Geometry check sheet. Reference: the model listing, model coordinates, mm. Face numbers are marked on the shaded views. Round coordinates to 2 decimals unless told otherwise and drop trailing zeros. Loops run counter-clockwise (first coordinate to the right, second up) from the corner with the lowest first, then second, coordinate; pieces in that order, holes last. Notation, with made-up numbers: (62, 48.5) -> (118, 48.5) arc R17 cw to (118, 70.5) -> close; hole circle Ø11 at (-35.5, 61). An arc over 180 degrees is marked (long way). Use a Markdown table: item, result. Add a question column.
Q1. Material ranges on L1, parallel to Y at x = 26, z = 5; L2, parallel to Y at x = 22, z = 6.25; L3, parallel to Y at x = 16, z = 0.75, recorded low to high.
Q2. Sectioned sample at D-D, the plane x = 11. Enter the section's corners in (y, z).
Q3. Sectioned sample at C-C, the plane y = -13. Enter the section's corners in (x, z).
Q4. Sectioned sample at A-A, the plane x = 0. Enter the section's corners in (y, z).
Q5. Gauge pin test, flat ends, axial feed: P1, Ø3.5, axis at x = 0, z = 4, coming from the +Y side; P2, Ø2.5, axis at x = -0.5, z = 3.5, coming from the -Y side; P3, Ø6, axis at x = -23.08, y = -23.08, coming from the +Z side. Record the tip position at first contact, or that the pin passes through.
Q6. Release check for a two-part mould opening along X. For the marked faces 1 and 2 record: released by +X, released by -X, zero draft, split by the parting line, or undercut.
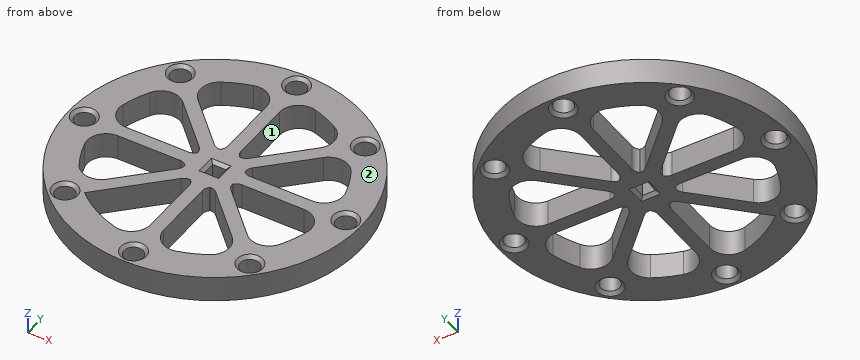
```python
from build123d import *

# Parameters (mm, degrees)
SKETCH1_R           = 36.449
SKETCH1_W           = 3.302
SKETCH1_H           = 3.302
SKETCH1_R_2         = 2.38125
BOSS_EXTRUDE1_DEPTH = 6.35
FILLET1_R           = 4.7625
FILLET2_R           = 2.38125
CHAMFER1_SIZE       = 0.79375


with BuildPart() as part:
    # Sketch1 → Boss-Extrude1 (new body)
    with BuildSketch(Plane.XY):
        Circle(SKETCH1_R)
        with BuildLine():
            Line((-1.651, 28.781685844), (-1.651, 6.131614714))
            ThreePointArc((-1.651, 6.131614714), (-2.430039796, 5.866635031), (-3.168273048, 5.50313964))
            Line((-3.168273048, 5.50313964), (-19.184291938, 21.51915853))
            ThreePointArc((-19.184291938, 21.51915853), (-11.032380672, 26.634523043), (-1.651, 28.781685844))
        make_face(mode=Mode.SUBTRACT)
        with BuildLine():
            Line((-21.51915853, 19.184291938), (-5.50313964, 3.168273048))
            ThreePointArc((-5.50313964, 3.168273048), (-5.866635031, 2.430039796), (-6.131614714, 1.651))
            Line((-6.131614714, 1.651), (-28.781685844, 1.651))
            ThreePointArc((-28.781685844, 1.651), (-26.634523043, 11.032380672), (-21.51915853, 19.184291938))
        make_face(mode=Mode.SUBTRACT)
        with BuildLine():
            Line((-28.781685844, -1.651), (-6.131614714, -1.651))
            ThreePointArc((-6.131614714, -1.651), (-5.866635031, -2.430039796), (-5.50313964, -3.168273048))
            Line((-5.50313964, -3.168273048), (-21.51915853, -19.184291938))
            ThreePointArc((-21.51915853, -19.184291938), (-26.634523043, -11.032380672), (-28.781685844, -1.651))
        make_face(mode=Mode.SUBTRACT)
        with BuildLine():
            Line((-19.184291938, -21.51915853), (-3.168273048, -5.50313964))
            ThreePointArc((-3.168273048, -5.50313964), (-2.430039796, -5.866635031), (-1.651, -6.131614714))
            Line((-1.651, -6.131614714), (-1.651, -28.781685844))
            ThreePointArc((-1.651, -28.781685844), (-11.032380672, -26.634523043), (-19.184291938, -21.51915853))
        make_face(mode=Mode.SUBTRACT)
        with BuildLine():
            Line((1.651, -28.781685844), (1.651, -6.131614714))
            ThreePointArc((1.651, -6.131614714), (2.430039796, -5.866635031), (3.168273048, -5.50313964))
            Line((3.168273048, -5.50313964), (19.184291938, -21.51915853))
            ThreePointArc((19.184291938, -21.51915853), (11.032380672, -26.634523043), (1.651, -28.781685844))
        make_face(mode=Mode.SUBTRACT)
        with BuildLine():
            Line((21.51915853, -19.184291938), (5.50313964, -3.168273048))
            ThreePointArc((5.50313964, -3.168273048), (5.866635031, -2.430039796), (6.131614714, -1.651))
            Line((6.131614714, -1.651), (28.781685844, -1.651))
            ThreePointArc((28.781685844, -1.651), (26.634523043, -11.032380672), (21.51915853, -19.184291938))
        make_face(mode=Mode.SUBTRACT)
        with BuildLine():
            Line((28.781685844, 1.651), (6.131614714, 1.651))
            ThreePointArc((6.131614714, 1.651), (5.866635031, 2.430039796), (5.50313964, 3.168273048))
            Line((5.50313964, 3.168273048), (21.51915853, 19.184291938))
            ThreePointArc((21.51915853, 19.184291938), (26.634523043, 11.032380672), (28.781685844, 1.651))
        make_face(mode=Mode.SUBTRACT)
        with BuildLine():
            Line((19.184291938, 21.51915853), (3.168273048, 5.50313964))
            ThreePointArc((3.168273048, 5.50313964), (2.430039796, 5.866635031), (1.651, 6.131614714))
            Line((1.651, 6.131614714), (1.651, 28.781685844))
            ThreePointArc((1.651, 28.781685844), (11.032380672, 26.634523043), (19.184291938, 21.51915853))
        make_face(mode=Mode.SUBTRACT)
        Rectangle(SKETCH1_W, SKETCH1_H, mode=Mode.SUBTRACT)
        with Locations((-23.079258231, -23.079258231)):
            Circle(SKETCH1_R_2, mode=Mode.SUBTRACT)
        with Locations((-32.639, 0)):
            Circle(SKETCH1_R_2, mode=Mode.SUBTRACT)
        with Locations((0, -32.639)):
            Circle(SKETCH1_R_2, mode=Mode.SUBTRACT)
        with Locations((23.079258231, -23.079258231)):
            Circle(SKETCH1_R_2, mode=Mode.SUBTRACT)
        with Locations((-23.079258231, 23.079258231)):
            Circle(SKETCH1_R_2, mode=Mode.SUBTRACT)
        with Locations((23.079258231, 23.079258231)):
            Circle(SKETCH1_R_2, mode=Mode.SUBTRACT)
        with Locations((0, 32.639)):
            Circle(SKETCH1_R_2, mode=Mode.SUBTRACT)
        with Locations((32.639, 0)):
            Circle(SKETCH1_R_2, mode=Mode.SUBTRACT)
    extrude(amount=BOSS_EXTRUDE1_DEPTH)

    # Fillet1
    fillet1_edges = [part.edges().sort_by_distance(p)[0] for p in [
        (21.51915853, 19.184291938, 3.175),
        (28.781685844, 1.651, 3.175),
        (19.184291938, 21.51915853, 3.175),
        (1.651, 28.781685844, 3.175),
        (-1.651, 28.781685844, 3.175),
        (-19.184291938, 21.51915853, 3.175),
        (-21.51915853, 19.184291938, 3.175),
        (-28.781685844, 1.651, 3.175),
        (-28.781685844, -1.651, 3.175),
        (-21.51915853, -19.184291938, 3.175),
        (-1.651, -28.781685844, 3.175),
        (1.651, -28.781685844, 3.175),
        (19.184291938, -21.51915853, 3.175),
        (21.51915853, -19.184291938, 3.175),
        (28.781685844, -1.651, 3.175),
    ]]
    fillet(fillet1_edges, radius=FILLET1_R)

    # Fillet2
    # the kernel refuses this fillet: 2.38125 mm, written as the material it adds along each edge
    with BuildSketch(Plane(origin=(6.131614714, -1.651, 0), x_dir=(-0.36304434778587014, -0.931771861316241, 0), z_dir=(0, 0, 1)), Plane(origin=(1.651, 6.131614714, 0), x_dir=(0.9317718613162208, -0.36304434778592154, 0), z_dir=(0, 0, 1)), Plane(origin=(5.50313964, 3.168273048, 0), x_dir=(0.40215108146465606, -0.9155733218463759, 0), z_dir=(0, 0, 1)), Plane(origin=(-6.131614714, 1.651, 0), x_dir=(0.3630443477859294, 0.9317718613162179, 0), z_dir=(0, 0, 1))) as fillet2_piece_1:
        with BuildLine():
            CenterArc((1.633270214, 2.367244602), FILLET2_R, 201.287277983, 62.495506179)
            Line((-0.585511531, 1.502745249), (0, 0))
            ThreePointArc((0, 0), (0.687692722, 0.037347727), (1.375385443, 0))
        make_face()
    extrude(amount=6.35)
    with BuildSketch(Plane(origin=(5.50313964, -3.168273048, 0), x_dir=(0.7071067811865454, -0.7071067811865497, 0), z_dir=(0, 0, 1)), Plane(origin=(3.168273048, 5.50313964, 0), x_dir=(0.7071067811865503, 0.7071067811865448, 0), z_dir=(0, 0, 1)), Plane(origin=(6.131614714, 1.651, 0), x_dir=(1, 0, 0), z_dir=(0, 0, 1)), Plane(origin=(-1.651, 6.131614714, 0), x_dir=(0, 1, 0), z_dir=(0, 0, 1)), Plane(origin=(-5.50313964, 3.168273048, 0), x_dir=(-0.7071067811865499, 0.7071067811865452, 0), z_dir=(0, 0, 1)), Plane(origin=(-6.131614714, -1.651, 0), x_dir=(-1, 0, 0), z_dir=(0, 0, 1)), Plane(origin=(1.651, -6.131614714, 0), x_dir=(0, -1, 0), z_dir=(0, 0, 1))) as fillet2_piece_2:
        with BuildLine():
            CenterArc((1.61278239, 2.38125), FILLET2_R, 207.504493821, 62.495506179)
            ThreePointArc((-0.499325911, 1.281545455), (-0.214863395, 0.654331608), (0, 0))
            Line((0, 0), (1.61278239, 0))
        make_face()
    extrude(amount=6.35)
    with BuildSketch(Plane(origin=(3.168273048, -5.50313964, 0), x_dir=(0.7071067811865439, -0.7071067811865511, 0), z_dir=(0, 0, 1)), Plane(origin=(-3.168273048, 5.50313964, 0), x_dir=(-0.7071067811865503, 0.7071067811865448, 0), z_dir=(0, 0, 1)), Plane(origin=(-5.50313964, -3.168273048, 0), x_dir=(-0.7071067811865455, -0.7071067811865496, 0), z_dir=(0, 0, 1)), Plane(origin=(-1.651, -6.131614714, 0), x_dir=(0, -1, 0), z_dir=(0, 0, 1))) as fillet2_piece_3:
        with BuildLine():
            CenterArc((1.61278239, -2.38125), FILLET2_R, 90, 62.495506179)
            ThreePointArc((-0.499325911, -1.281545455), (-0.214863395, -0.654331608), (0, 0))
            Line((0, 0), (1.61278239, 0))
        make_face()
    extrude(amount=6.35)
    with BuildSketch(Plane(origin=(-3.168273048, -5.50313964, 0), x_dir=(0.9155733218463795, -0.40215108146464806, 0), z_dir=(0, 0, 1))) as fillet2_piece_4:
        with BuildLine():
            CenterArc((1.633270214, -2.367244602), FILLET2_R, 96.217215838, 62.495506179)
            Line((-0.585511531, -1.502745249), (0, 0))
            ThreePointArc((0, 0), (0.687692722, -0.037347727), (1.375385443, 0))
        make_face()
    extrude(amount=6.35)

    # Chamfer1
    chamfer1_edges = [part.edges().sort_by_distance(p)[0] for p in [
        (-25.460508231, 23.079258231, 6.35),
        (-35.02025, 0, 6.35),
        (-25.460508231, -23.079258231, 6.35),
        (-2.38125, -32.639, 6.35),
        (20.698008231, -23.079258231, 6.35),
        (30.25775, 0, 6.35),
        (20.698008231, 23.079258231, 6.35),
        (-2.38125, 32.639, 6.35),
        (0, -1.651, 6.35),
        (-1.651, 0, 6.35),
        (0, 1.651, 6.35),
        (1.651, 0, 6.35),
        (1.651, 0, 0),
        (0, 1.651, 0),
        (-1.651, 0, 0),
        (0, -1.651, 0),
        (-2.38125, 32.639, 0),
        (20.698008231, 23.079258231, 0),
        (30.25775, 0, 0),
        (20.698008231, -23.079258231, 0),
        (-2.38125, -32.639, 0),
        (-25.460508231, -23.079258231, 0),
        (-35.02025, 0, 0),
        (-25.460508231, 23.079258231, 0),
    ]]
    chamfer(chamfer1_edges, length=CHAMFER1_SIZE)


solid = part.part
```
Values:
| question | item | result |
|---|---|---|
| 1 | L1 | -25.54 to -12.45, -2.56 to 2.56, 12.45 to 25.54 |
| 1 | L2 | -29.06 to -25.96, -20.2 to -16.51, -1.65 to 1.65, 16.51 to 20.2, 25.96 to 29.06 |
| 1 | L3 | -32.75 to -23.3, -18.57 to -13.67, -1.65 to 1.65, 13.67 to 18.57, 23.3 to 32.75 |
| 2 | outline | (-34.75, 0) -> (-26.65, 0) -> (-26.65, 6.35) -> (-34.75, 6.35) -> close; (-13.33, 0) -> (-8.67, 0) -> (-8.67, 6.35) -> (-13.33, 6.35) -> close; (-1.65, 0) -> (1.65, 0) -> (1.65, 6.35) -> (-1.65, 6.35) -> close; (8.67, 0) -> (13.33, 0) -> (13.33, 6.35) -> (8.67, 6.35) -> close; (26.65, 0) -> (34.75, 0) -> (34.75, 6.35) -> (26.65, 6.35) -> close |
| 3 | outline | (-34.05, 0) -> (-25.73, 0) -> (-25.73, 6.35) -> (-34.05, 6.35) -> close; (-15.33, 0) -> (-10.67, 0) -> (-10.67, 6.35) -> (-15.33, 6.35) -> close; (-1.65, 0) -> (1.65, 0) -> (1.65, 6.35) -> (-1.65, 6.35) -> close; (10.67, 0) -> (15.33, 0) -> (15.33, 6.35) -> (10.67, 6.35) -> close; (25.73, 0) -> (34.05, 0) -> (34.05, 6.35) -> (25.73, 6.35) -> close |
| 4 | outline | (-36.45, 0) -> (-35.81, 0) -> (-35.02, 0.79) -> (-35.02, 5.56) -> (-35.81, 6.35) -> (-36.45, 6.35) -> close; (-30.26, 0.79) -> (-29.46, 0) -> (-2.44, 0) -> (-1.65, 0.79) -> (-1.65, 5.56) -> (-2.44, 6.35) -> (-29.46, 6.35) -> (-30.26, 5.56) -> close; (1.65, 0.79) -> (2.44, 0) -> (29.46, 0) -> (30.26, 0.79) -> (30.26, 5.56) -> (29.46, 6.35) -> (2.44, 6.35) -> (1.65, 5.56) -> close; (35.02, 0.79) -> (35.81, 0) -> (36.45, 0) -> (36.45, 6.35) -> (35.81, 6.35) -> (35.02, 5.56) -> close |
| 5 | P1 | y = 36.45 |
| 5 | P2 | y = -36.45 |
| 5 | P3 | z = 6.18 |
| 6 | face 1 | undercut |
| 6 | face 2 | zero draft |
